Build history of the part. All positions in model axes, mm. Face numbers are marked on the shaded views. A direction names the side the tool comes from. Coordinates: 2 decimals unless noted, no trailing zeros. Loops run counter-clockwise (first coordinate to the right, second up) from the corner with the lowest first, then second, coordinate; pieces in that order, holes last.
Item 1: Cut at A-A (z = 233.5). List the corners of the cut face in (x, y).
Item 2: Cut at B-B (x = -431.8). List the corners of the cut face in (y, z).
Item 3: Cut at D-D (y = -177.8). List the corners of the cut face in (x, z).
Item 4: Mould opens along X. For the marked faces 3, 4, 5 and 6 say: released by +X, released by -X, zero draft, split by the parting line, or undercut.
Item 5: Cut at C-C (y = -98.5). List the corners of the cut face in (x, z).
Item 6: 3-axis set-ups, long thin cutter, end or side, ignore diameter. For the marked faces 1 and 2: which of +Z, -Z, +X, -X, +Y, -Y reach the whole face in a straight line?
Item 7: Drill centre lines: line 1 along Z through (x, y) = (-231, -79.5); line 2 along Y through (x, z) = (-464.5, 240); line 3 along X through (y, z) = (-144, 227). Where is each one in solid material? Low to high.
from build123d import *

# Parameters (mm, degrees)
F0_W     = 1016
F0_H     = 508
F1_DEPTH = 368.3
F2_W     = 330.2
F2_H     = 330.2
F3_DEPTH = 177.8
F4_R     = 25.4
F5_DEPTH = 101.6


with BuildPart() as f1:
    # F0 (on Top) → F1 (new body)
    with BuildSketch(Plane.XY):
        Rectangle(F0_W, F0_H)
    extrude(amount=F1_DEPTH)

    # F2 (on face) → F3 (cut)
    with BuildSketch(Plane.XY.offset(368.3)):
        with Locations((-342.9, -88.9)):
            Rectangle(F2_W, F2_H)
    extrude(amount=-F3_DEPTH, mode=Mode.SUBTRACT)

    # F4 (on face) → F5 (join)
    with BuildSketch(Plane.XY.offset(190.5)):
        with Locations((-431.8, -177.8)):
            Circle(F4_R)
    extrude(amount=F5_DEPTH)


solid = f1.part
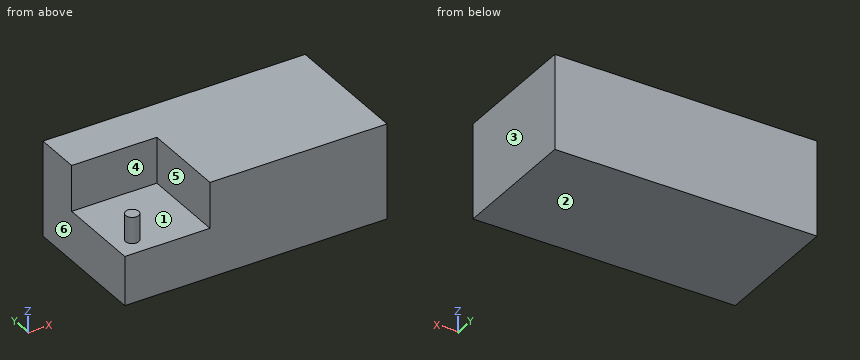
Filled sheet:
1. outline: (-508, 76.2) - (-177.8, 76.2) - (-177.8, -254) - (508, -254) - (508, 254) - (-508, 254) - close; circle Ø50.8 at (-431.8, -177.8)
2. outline: (-254, 0) - (254, 0) - (254, 368.3) - (76.2, 368.3) - (76.2, 190.5) - (-152.4, 190.5) - (-152.4, 292.1) - (-203.2, 292.1) - (-203.2, 190.5) - (-254, 190.5) - close
3. outline: (-508, 0) - (508, 0) - (508, 368.3) - (-177.8, 368.3) - (-177.8, 190.5) - (-406.4, 190.5) - (-406.4, 292.1) - (-457.2, 292.1) - (-457.2, 190.5) - (-508, 190.5) - close
4. face 3: released by +X
4. face 4: zero draft
4. face 5: undercut
4. face 6: released by -X
5. outline: (-508, 0) - (508, 0) - (508, 368.3) - (-177.8, 368.3) - (-177.8, 190.5) - (-508, 190.5) - close
6. face 1: +Z
6. face 2: -Z, +X, -X, +Y, -Y
7. line 1: z = 0 to 190.5
7. line 2: y = 76.2 to 254
7. line 3: x = -177.8 to 508
